```python
from build123d import *

# Parameters (mm, degrees)
F1_DEPTH = 14.5
F3_DEPTH = 6.6
F4_R     = 1
F5_R     = 2.25
F6_DEPTH = 10.2
F7_R     = 1.75
F8_DEPTH = 25


with BuildPart() as f1:
    # F0 (on Top) → F1 (new body)
    with BuildSketch(Plane.XY):
        with BuildLine():
            ThreePointArc((1.75, -2.8), (4.55, 0), (1.75, 2.8))
            Line((1.75, 2.8), (-1.75, 2.8))
            ThreePointArc((-1.75, 2.8), (-4.55, 0), (-1.75, -2.8))
            Line((-1.75, -2.8), (1.75, -2.8))
        make_face()
    extrude(amount=F1_DEPTH)

    # F2 (on face) → F3 (join)
    with BuildSketch(Plane.XY.offset(14.5)):
        with BuildLine():
            Line((3.264966, 0.75), (-3.264966, 0.75))
            ThreePointArc((-3.264966, 0.75), (-3.35, 0), (-3.264966, -0.75))
            Line((-3.264966, -0.75), (3.264966, -0.75))
            ThreePointArc((3.264966, -0.75), (3.35, 0), (3.264966, 0.75))
        make_face()
    extrude(amount=F3_DEPTH)

    # F4
    f4_edges = [f1.edges().sort_by_distance(p)[0] for p in [
        (-3.35, 0, 21.1),
        (3.35, 0, 21.1),
    ]]
    fillet(f4_edges, radius=F4_R)

    # F5 (on face) → F6 (join)
    with BuildSketch(Plane(origin=(0, 0, 0), x_dir=(1, 0, 0), z_dir=(0, 0, -1))):
        Circle(F5_R)
    extrude(amount=F6_DEPTH)

    # F7 (on face) → F8 (join)
    with BuildSketch(Plane(origin=(0, 0, -10.2), x_dir=(1, 0, 0), z_dir=(0, 0, -1))):
        Circle(F7_R)
    extrude(amount=F8_DEPTH)


solid = f1.part
```
For this review, take the finished solid that the model builds, in its own axes (mm). A direction names the side the tool comes from. Give positions to 0.01 mm unless a question says otherwise; leave off trailing zeros. Order: outer loops, then holes, each group sorted by start corner. A loop starts at its lowest first (then second) coordinate and runs counter-clockwise, first axis right, second up.
1) Wall thickness on line 1 (Z direction, x = -1.5, y = 1.85); line 2 (Z direction, x = -0.75, y = 1.5); line 3 (X direction, y = -0.2, z = -24): over which ranges is each line inside the solid? List them lowest first.
2) Take a section at C-C (z = 16). Give the boundary of the cut face in (x, y).
3) For faces 1 (the face through (-3.35, 0.01, 17.26)), 2 (the face through (1.617, 0.67, -22.525)), 3 (the face through (0, 0.75, 18)), 4 (the face through (0, -0.75, 18)), list the 3-axis set-ups (+Z, -Z, +X, -X, +Y, -Y) from which the entire face can be reached by the end or side of a thin tool; tool diameter is ignored.
4) Take a section at A-A (y = 0). Give the boundary of the cut face in (x, z), then the cut area to 3 significant figures.
5) Take a section at B-B (x = 0). Give the boundary of the cut face in (y, z), then the cut area to 4 significant figures.
6) Insertion check: pin 1 (3.5 mm diameter, centred on x = -1, z = 17.5, fed in from -Y); pin 2 (5 mm diameter, centred on x = -1, z = 18, fed in from +Y); pin 3 (3 mm diameter, centred on x = 1.5, y = -1, fed in from -Z); pin 4 (1.5 mm diameter, centred on x = 3.5, y = -1.5, fed in from -Z). Each pin has a flat end and moves straight along its axis. Give the tip position at first contact, or say it passes through.
7) Take a section at D-D (z = -6). Give the boundary of the cut face in (x, y).
Derived:
1. line 1: z = 0 to 14.5
1. line 2: z = -35.2 to 14.5
1. line 3: x = -1.74 to 1.74
2. outline: (-3.26, -0.75) - (3.26, -0.75) arc R3.35 ccw to (3.26, 0.75) - (-3.26, 0.75) arc R3.35 ccw to start
3. face 1: +Z, -X
3. face 2: -Z
3. face 3: +Z, +X, -X, +Y
3. face 4: +Z, +X, -X, -Y
4. outline: (-4.55, 0) - (-2.25, 0) - (-2.25, -10.2) - (-1.75, -10.2) - (-1.75, -35.2) - (1.75, -35.2) - (1.75, -10.2) - (2.25, -10.2) - (2.25, 0) - (4.55, 0) - (4.55, 14.5) - (3.35, 14.5) - (3.35, 20.1) arc R1 ccw to (2.35, 21.1) - (-2.35, 21.1) arc R1 ccw to (-3.35, 20.1) - (-3.35, 14.5) - (-4.55, 14.5) - close
4. area: 309 mm2
5. outline: (-2.8, 0) - (-2.25, 0) - (-2.25, -10.2) - (-1.75, -10.2) - (-1.75, -35.2) - (1.75, -35.2) - (1.75, -10.2) - (2.25, -10.2) - (2.25, 0) - (2.8, 0) - (2.8, 14.5) - (0.75, 14.5) - (0.75, 21.1) - (-0.75, 21.1) - (-0.75, 14.5) - (-2.8, 14.5) - close
5. area: 224.5 mm2
6. pin 1: stops at y = -0.75
6. pin 2: stops at y = 0.75
6. pin 3: stops at z = -35.2
6. pin 4: stops at z = 0
7. outline: circle Ø4.5 at (0, 0)
